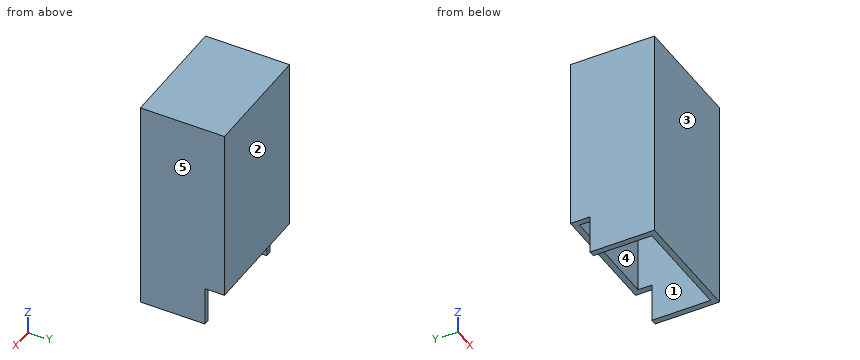
from build123d import *

# Parameters (mm, degrees)
IZIM1_W                     = 60
IZIM1_H                     = 43.037715622
IZIM1_W_2                   = 54
IZIM1_H_2                   = 37.037715622
Y_KSEKLIK_EKSTR_ZYON1_DEPTH = 110
IZIM2_W                     = 60
IZIM2_H                     = 20
KES_EKSTR_ZYON1_DEPTH       = 10
IZIM3_W                     = 60
IZIM3_H                     = 43.037715622
Y_KSEKLIK_EKSTR_ZYON2_DEPTH = 10


with BuildPart() as part:
    # Çizim1 → Yükseklik-Ekstrüzyon1 (new body)
    with BuildSketch(Plane.XY):
        with Locations((30, 21.518857811)):
            Rectangle(IZIM1_W, IZIM1_H)
        with Locations((30, 21.518857811)):
            Rectangle(IZIM1_W_2, IZIM1_H_2, mode=Mode.SUBTRACT)
    extrude(amount=Y_KSEKLIK_EKSTR_ZYON1_DEPTH)

    # Çizim2 → Kes-Ekstrüzyon1 (cut)
    with BuildSketch(Plane(origin=(0, 43.037715622, 0), x_dir=(1, 0, 0), z_dir=(0, 1, 0))):
        with Locations((30, -10)):
            Rectangle(IZIM2_W, IZIM2_H)
    extrude(amount=-KES_EKSTR_ZYON1_DEPTH, mode=Mode.SUBTRACT)

    # Çizim3 → Yükseklik-Ekstrüzyon2 (add)
    with BuildSketch(Plane.XY.offset(110)):
        with Locations((30, 21.518857811)):
            Rectangle(IZIM3_W, IZIM3_H)
    extrude(amount=-Y_KSEKLIK_EKSTR_ZYON2_DEPTH)


solid = part.part
Could you check a few things on this model? Use its own coordinates, in mm. Face numbers are marked on the shaded views. A direction names the side the tool comes from. Coordinates: 2 decimals unless noted, no trailing zeros. Loops run counter-clockwise (first coordinate to the right, second up) from the corner with the lowest first, then second, coordinate; pieces in that order, holes last.
1. Imagine slicing it at C-C (y = 8.5). Please give me the cut outline in (x, z).
2. Imagine slicing it at A-A (z = 57). Please give me the cut outline in (x, y), and give its area (3 significant figures).
3. We'd pull the mould along X, two halves only. Please class the marked faces 3, 4 and 5: released by +X, released by -X, zero draft, split by the parting line, or undercut.
4. For P1, Ø1.5, axis at x = 59, z = 14, coming from the +Y side; P2, Ø1.5, axis at x = 8.5, y = 30, coming from the -Z side; P3, Ø11, axis at x = 33, y = 38.5, coming from the -Z side, each with a flat end and sliding along its axis, tell me the tip position at first contact or that it passes through.
5. For the marked faces 1 and 2, which set-ups out of +Z, -Z, +X, -X, +Y, -Y let a thin tool reach every point of the face, with its end or its side?
6. Imagine slicing it at B-B (x = 6). Please give me the cut outline in (y, z).
7. I need wall thicknesses on L1, parallel to X at y = 9.5, z = 13; L2, parallel to Y at x = 44, z = 25; L3, parallel to Z at x = 32.5, y = 18. Which ranges of each line are inside material? Lowest first, please.
Computed values:
1. outline: (0, 0) - (3, 0) - (3, 100) - (57, 100) - (57, 0) - (60, 0) - (60, 110) - (0, 110) - close
2. outline: (0, 0) - (60, 0) - (60, 43.04) - (0, 43.04) - close; hole (3, 3) - (57, 3) - (57, 40.04) - (3, 40.04) - close
2. area: 582 mm2
3. face 3: zero draft
3. face 4: undercut
3. face 5: released by +X
4. P1: stops at y = 33.04
4. P2: stops at z = 100
4. P3: stops at z = 20
5. face 1: -Z
5. face 2: +Z, -Z, +X, -X, +Y
6. outline: (0, 0) - (3, 0) - (3, 100) - (40.04, 100) - (40.04, 20) - (43.04, 20) - (43.04, 110) - (0, 110) - close
7. L1: x = 0 to 3, 57 to 60
7. L2: y = 0 to 3, 40.04 to 43.04
7. L3: z = 100 to 110
